Geometry check sheet. Reference: drawing and pictorial views, mm from the part's lowest x, y, z. Round coordinates to 2 decimals unless told otherwise and drop trailing zeros. Write each loop counter-clockwise with the first axis right and the second up, starting at its lowest first coordinate (ties: lowest second). Pieces come first, ordered by that corner, then holes. Notation, with made-up numbers: (-32.5, -7.75) -> (-5.5, -7.75) arc R23 ccw to (-5.5, 19.25) -> close; hole circle Ø3 at (47.5, 39.5). An arc over 180 degrees is marked (long way). Answer as a JSON object with one key per item and string values. Group by question number.
(1) Sectioned sample at C-C on z = 1.6. Count the separate pieces of the cut face and the enclosed holes in it, and give its area (3 significant figures).
(2) Gauge pin test, flat end, axial feed: pin 1 Ø3 at (x, y) = (72.5, 20) entering from -Z. Record the tip position at first contact, or that the pin passes through.
(3) Sectioned sample at A-A on y = 30. Record the cut outline in (x, z), and give its area (3 significant figures).
(4) Sectioned sample at B-B on x = 40. Record the cut outline in (y, z).
(5) Scan lines: L1, parallel to Y at x = 7.5, z = 2.15; L2, parallel to X at y = 20, z = 2.1; L3, parallel to X at y = 31, z = 0.6. Record each from-to range of solid material in increasing order. Write a range as from..to.
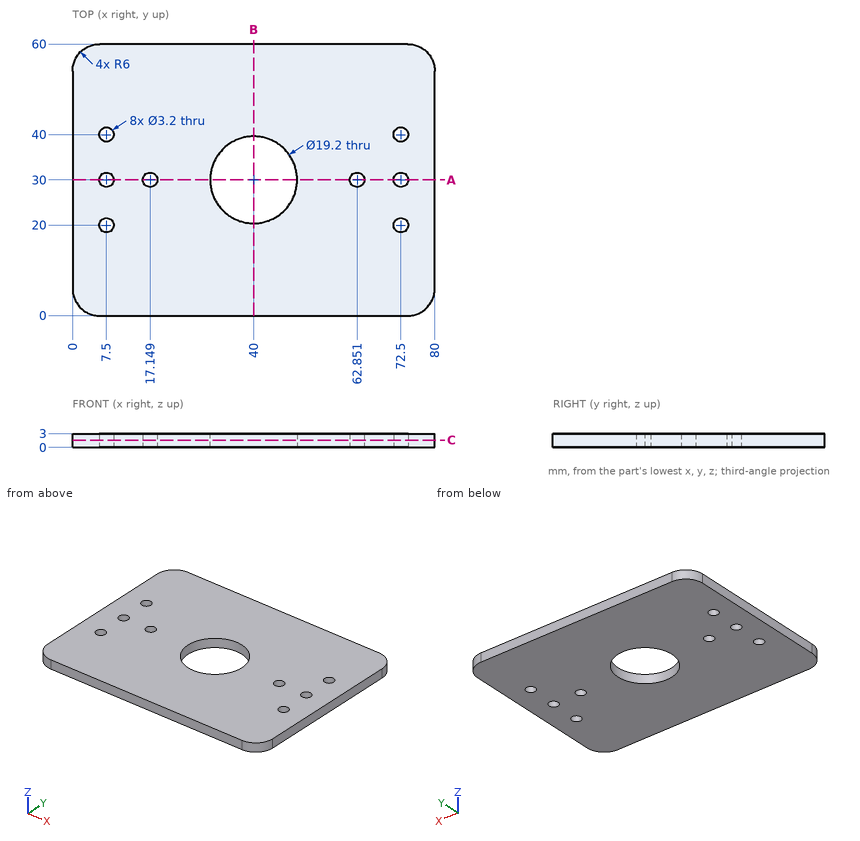
Computed values:
{
 "1": {"separate pieces": "1", "enclosed holes": "9", "area": "4,420 mm2"},
 "2": {"pin 1": "through"},
 "3": {"outline": "(0, 0) -> (5.9, 0) -> (5.9, 3) -> (0, 3) -> close; (9.1, 0) -> (15.55, 0) -> (15.55, 3) -> (9.1, 3) -> close; (18.75, 0) -> (30.4, 0) -> (30.4, 3) -> (18.75, 3) -> close; (49.6, 0) -> (61.25, 0) -> (61.25, 3) -> (49.6, 3) -> close; (64.45, 0) -> (70.9, 0) -> (70.9, 3) -> (64.45, 3) -> close; (74.1, 0) -> (80, 0) -> (80, 3) -> (74.1, 3) -> close", "area": "144 mm2"},
 "4": {"outline": "(0, 0) -> (20.4, 0) -> (20.4, 3) -> (0, 3) -> close; (39.6, 0) -> (60, 0) -> (60, 3) -> (39.6, 3) -> close"},
 "5": {"L1": "0..18.4, 21.6..28.4, 31.6..38.4, 41.6..60", "L2": "0..5.9, 9.1..70.9, 74.1..80", "L3": "0..6.25, 8.75..15.9, 18.4..30.45, 49.55..61.6, 64.1..71.25, 73.75..80"}
}
